from build123d import *

# Parameters (mm, degrees)
ESQUISSE1_R             = 125
BOSS_EXTRU_1_DEPTH      = 15
ESQUISSE2_R             = 7.5
ESQUISSE2_R_2           = 5
ESQUISSE2_W             = 15
ESQUISSE2_H             = 15
ESQUISSE2_W_2           = 28.64
ESQUISSE2_H_2           = 18.12
ESQUISSE2_W_3           = 45
ENL_V_MAT_EXTRU_1_DEPTH = 178.411949992


with BuildPart() as part:
    # Esquisse1 → Boss.-Extru.1 (new body)
    with BuildSketch(Plane.XY):
        Circle(ESQUISSE1_R)
    extrude(amount=BOSS_EXTRU_1_DEPTH)

    # Esquisse2 → Enlèv. mat.-Extru.1 (cut, through all)
    with BuildSketch(Plane.XY.offset(15)):
        Circle(ESQUISSE2_R)
        with Locations((47.610253526, 44.194173824)):
            Circle(ESQUISSE2_R_2)
        with Locations((-47.610253526, 44.194173824)):
            Circle(ESQUISSE2_R_2)
        with Locations((70.110253526, 44.194173824)):
            Rectangle(ESQUISSE2_W, ESQUISSE2_H)
        with Locations((-70.110253526, 44.194173824)):
            Rectangle(ESQUISSE2_W, ESQUISSE2_H)
        with Locations((59.648339804, 0)):
            Rectangle(ESQUISSE2_W_2, ESQUISSE2_H_2)
        with Locations((-10.110253526, 44.194173824)):
            Rectangle(ESQUISSE2_W_3, ESQUISSE2_H)
    enl_v_mat_extru_1 = extrude(amount=-ENL_V_MAT_EXTRU_1_DEPTH, mode=Mode.SUBTRACT)

    # Symétrie1: Enlèv. mat.-Extru.1 across plane
    add(enl_v_mat_extru_1.mirror(Plane.ZX), mode=Mode.SUBTRACT)


solid = part.part
Build history of the part. All positions in model axes, mm. Coordinates: 2 decimals unless noted, no trailing zeros. Order: outer loops, then holes, each group sorted by start corner. A loop starts at its lowest first (then second) coordinate and runs counter-clockwise, first axis right, second up. Notation, with made-up numbers: (40, 88.5) -> (99, 88.5) arc R28 cw to (99, 115.5) -> close; hole circle Ø1 at (18.25, 22). An arc over 180 degrees is marked (long way). One line per item, written item: value.
(1) Probe line 1 (Y direction, x = 6, z = 3.5); line 2 (Y direction, x = -76.5, z = 8.5); line 3 (Y direction, x = -15.5, z = 4.5). List the from-to ranges inside material, lowest first. Write a range as [from, to].
Checked values:
line 1: [-124.86, -51.69], [-36.69, -4.5], [4.5, 36.69], [51.69, 124.86]
line 2: [-98.86, -51.69], [-36.69, 36.69], [51.69, 98.86]
line 3: [-124.04, -51.69], [-36.69, 36.69], [51.69, 124.04]
(2) Slice it at B-B, the plane x = 0. List the corners of the cut face in (y, z).
Checked values:
outline: (-125, 0) -> (-51.69, 0) -> (-51.69, 15) -> (-125, 15) -> close; (-36.69, 0) -> (-7.5, 0) -> (-7.5, 15) -> (-36.69, 15) -> close; (7.5, 0) -> (36.69, 0) -> (36.69, 15) -> (7.5, 15) -> close; (51.69, 0) -> (125, 0) -> (125, 15) -> (51.69, 15) -> close
(3) Slice it at C-C, the plane x = -48.5. List the corners of the cut face in (y, z), plus the area to 3 significant figures.
Checked values:
outline: (-115.21, 0) -> (-49.11, 0) -> (-49.11, 15) -> (-115.21, 15) -> close; (-39.27, 0) -> (39.27, 0) -> (39.27, 15) -> (-39.27, 15) -> close; (49.11, 0) -> (115.21, 0) -> (115.21, 15) -> (49.11, 15) -> close
area: 3,160 mm2
(4) Slice it at A-A, the plane y = 0. List the corners of the cut face in (x, z).
Checked values:
outline: (-125, 0) -> (-7.5, 0) -> (-7.5, 15) -> (-125, 15) -> close; (7.5, 0) -> (45.33, 0) -> (45.33, 15) -> (7.5, 15) -> close; (73.97, 0) -> (125, 0) -> (125, 15) -> (73.97, 15) -> close
(5) Mould opens along Y. For faces 1 (the flat face through (70, -51.694, 8)), 2 (the cylindrical face through (-48.694, -39.313, 7.605)) say: pulls with the +Y half, pulls with the -Y half, needs draft (parallel to the pull), parting line crosses it, or undercut.
Checked values:
face 1: undercut
face 2: undercut
(6) Drop flat-ended pins along their axis: pin 1 Ø3 at (x, z) = (-97.5, 5) entering from -Y; pin 2 Ø7.5 at (y, z) = (45.5, 11) entering from -X; pin 3 Ø7.5 at (y, z) = (-43, 10) entering from -X. Give the stop position or say it passes through.
Checked values:
pin 1: y = -80.06
pin 2: x = -117.82
pin 3: x = -118.68
(7) Slice it at D-D, the plane z = 8.25. Count the separate pieces of the cut face and the enclosed holes in it, plus the area to 3 significant figures.
Checked values:
separate pieces: 1
enclosed holes: 12
area: 45,800 mm2
